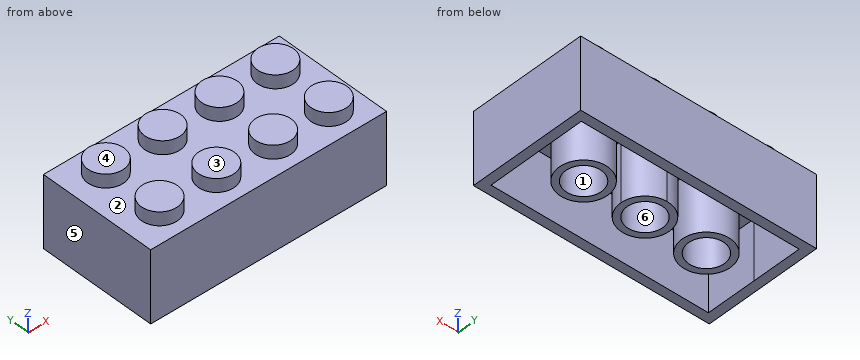
from build123d import *

# Parameters (mm, degrees)
F0_W     = 31.64
F0_H     = 15.74
F1_DEPTH = 9.59
F2_R     = 2.425
F3_DEPTH = 1.8
F5_DEPTH = 8


with BuildPart() as f1:
    # F0 (on Top) → F1 (new body)
    with BuildSketch(Plane.XY):
        with Locations((15.82, 7.87)):
            Rectangle(F0_W, F0_H)
    extrude(amount=F1_DEPTH)

    # F2 (on face) → F3 (join)
    with BuildSketch(Plane.XY.offset(9.59)):
        with Locations((4.7746349379, 11.815)):
            Circle(F2_R)
        with Locations((12.3955499551, 11.815)):
            Circle(F2_R)
        with Locations((20.0164649723, 11.815)):
            Circle(F2_R)
        with Locations((27.4894218309, 11.7763556091)):
            Circle(F2_R)
        with Locations((4.7746349379, 3.925)):
            Circle(F2_R)
        with Locations((12.3955499551, 3.925)):
            Circle(F2_R)
        with Locations((20.0164649723, 3.925)):
            Circle(F2_R)
        with Locations((27.4894218309, 3.925)):
            Circle(F2_R)
    extrude(amount=F3_DEPTH)

    # F4 (on face) → F5 (cut)
    with BuildSketch(Plane(origin=(0, 0, 0), x_dir=(1, 0, 0), z_dir=(0, 0, -1))):
        with BuildLine():
            ThreePointArc((19.07, -7.87), (18.1189275762, -10.1672662012), (15.8223495388, -11.1199991507))
            Line((15.8223495388, -11.1199991507), (15.8223495388, -14.52))
            Line((15.8223495388, -14.52), (30.4358961851, -14.52))
            Line((30.4358961851, -14.52), (30.4199965129, -7.87))
            Line((30.4199965129, -7.87), (27.31, -7.87))
            ThreePointArc((27.31, -7.87), (24.06, -11.12), (20.81, -7.87))
            Line((20.81, -7.87), (19.07, -7.87))
        make_face()
        with BuildLine():
            Line((15.817648704, -1.22), (15.817648704, -4.6200008506))
            ThreePointArc((15.817648704, -4.6200008506), (18.1172655798, -5.5710718028), (19.07, -7.87))
            Line((19.07, -7.87), (20.81, -7.87))
            ThreePointArc((20.81, -7.87), (24.06, -4.62), (27.31, -7.87))
            Line((27.31, -7.87), (30.4199965129, -7.87))
            Line((30.4199965129, -7.87), (30.4040968407, -1.22))
            Line((30.4040968407, -1.22), (15.817648704, -1.22))
        make_face()
        with BuildLine():
            ThreePointArc((4.33, -7.87), (7.58, -4.62), (10.83, -7.87))
            Line((10.83, -7.87), (12.57, -7.87))
            ThreePointArc((12.57, -7.87), (13.5210718028, -5.5727344202), (15.817648704, -4.6200008506))
            Line((15.817648704, -4.6200008506), (15.817648704, -1.22))
            Line((15.817648704, -1.22), (1.2312005673, -1.22))
            Line((1.2312005673, -1.22), (1.2200017299, -7.87))
            Line((1.2200017299, -7.87), (4.33, -7.87))
        make_face()
        with BuildLine():
            Line((12.57, -7.87), (10.83, -7.87))
            ThreePointArc((10.83, -7.87), (7.58, -11.12), (4.33, -7.87))
            Line((4.33, -7.87), (1.2200017299, -7.87))
            Line((1.2200017299, -7.87), (1.2088028926, -14.52))
            Line((1.2088028926, -14.52), (15.8223495388, -14.52))
            Line((15.8223495388, -14.52), (15.8223495388, -11.1199991507))
            ThreePointArc((15.8223495388, -11.1199991507), (13.5227337988, -10.1689275762), (12.57, -7.87))
        make_face()
        with BuildLine():
            Line((5.18, -7.87), (9.98, -7.87))
            ThreePointArc((9.98, -7.87), (7.58, -5.47), (5.18, -7.87))
        make_face()
        with BuildLine():
            ThreePointArc((5.18, -7.87), (7.58, -10.27), (9.98, -7.87))
            Line((9.98, -7.87), (5.18, -7.87))
        make_face()
        with BuildLine():
            Line((18.22, -7.87), (13.42, -7.87))
            ThreePointArc((13.42, -7.87), (15.82, -10.27), (18.22, -7.87))
        make_face()
        with BuildLine():
            ThreePointArc((18.22, -7.87), (15.82, -5.47), (13.42, -7.87))
            Line((13.42, -7.87), (18.22, -7.87))
        make_face()
        with BuildLine():
            ThreePointArc((26.46, -7.87), (24.06, -5.47), (21.66, -7.87))
            Line((21.66, -7.87), (26.46, -7.87))
        make_face()
        with BuildLine():
            Line((26.46, -7.87), (21.66, -7.87))
            ThreePointArc((21.66, -7.87), (24.06, -10.27), (26.46, -7.87))
        make_face()
    extrude(amount=-F5_DEPTH, mode=Mode.SUBTRACT)


solid = f1.part
Here's how the part is built. I have some questions about the finished solid (model axes, mm). Face numbers are marked on the shaded views. A direction names the side the tool comes from. Give positions to 0.01 mm unless a question says otherwise; leave off trailing zeros. Order: outer loops, then holes, each group sorted by start corner. A loop starts at its lowest first (then second) coordinate and runs counter-clockwise, first axis right, second up. Notation, with made-up numbers: (-16.75, 37) -> (30.25, 37) arc R16 ccw to (30.25, 41) -> close; hole circle Ø10 at (74.25, -10). An arc over 180 degrees is marked (long way). Use a Markdown table: item, result. Add a question column.
Item 1: If we mould it in two halves opening along X, with no side actions, what happens to the marked faces 4, 5 and 6? For each: pulls with the +X half, pulls with the -X half, needs draft (parallel to the pull), parting line crosses it, or undercut.
Item 2: I need wall thicknesses on line 1 (Y direction, x = 7.58, z = 5.75); line 2 (Y direction, x = 29, z = 1.75); line 3 (Y direction, x = 5, z = 0.5). Which ranges of each line are inside material? Lowest first, please.
Item 3: Imagine slicing it at C-C on y = 13. Please give me the cut outline in (x, z), plus the area to 3 significant figures.
Item 4: Will these pins go through, and if not, where does the flat tip stop? pin 1 (3 mm diameter, centred on x = 15.82, y = 7.87, fed in from +Z); pin 2 (2.5 mm diameter, centred on x = 8.5, y = 8, fed in from -Z).
Item 5: Imagine slicing it at B-B on x = 24.06. Please give me the cut outline in (y, z), plus the area to 3 significant figures.
Item 6: Imagine slicing it at A-A on z = 5.5. Please give me the cut outline in (x, y), plus the area to 3 significant figures.
Item 7: Imagine slicing it at D-D on x = 2. Please give me the cut outline in (y, z), plus the area to 3 significant figures.
Item 8: For the marked faces 1, 2 and 3, which set-ups out of +Z, -Z, +X, -X, +Y, -Y let a thin tool reach every point of the face, with its end or its side?
Data:
| question | item | result |
|---|---|---|
| 1 | face 4 | needs draft |
| 1 | face 5 | pulls with the -X half |
| 1 | face 6 | undercut |
| 2 | line 1 | y = 0 to 1.22, 4.62 to 5.47, 10.27 to 11.12, 14.52 to 15.74 |
| 2 | line 2 | y = 0 to 1.22, 14.52 to 15.74 |
| 2 | line 3 | y = 0 to 1.22, 5.89 to 9.85, 14.52 to 15.74 |
| 3 | outline | (0, 0) -> (1.21, 0) -> (1.21, 8) -> (30.43, 8) -> (30.43, 0) -> (31.64, 0) -> (31.64, 9.59) -> (29.58, 9.59) -> (29.58, 11.39) -> (25.4, 11.39) -> (25.4, 9.59) -> (22.13, 9.59) -> (22.13, 11.39) -> (17.9, 11.39) -> (17.9, 9.59) -> (14.51, 9.59) -> (14.51, 11.39) -> (10.28, 11.39) -> (10.28, 9.59) -> (6.89, 9.59) -> (6.89, 11.39) -> (2.66, 11.39) -> (2.66, 9.59) -> (0, 9.59) -> close |
| 3 | area | 100 mm² |
| 4 | pin 1 | stops at z = 9.59 |
| 4 | pin 2 | stops at z = 8 |
| 5 | outline | (0, 0) -> (1.22, 0) -> (1.22, 8) -> (4.62, 8) -> (4.62, 0) -> (5.47, 0) -> (5.47, 8) -> (10.27, 8) -> (10.27, 0) -> (11.12, 0) -> (11.12, 8) -> (14.52, 8) -> (14.52, 0) -> (15.74, 0) -> (15.74, 9.59) -> (0, 9.59) -> close |
| 5 | area | 58.1 mm² |
| 6 | outline | (0, 0) -> (31.64, 0) -> (31.64, 15.74) -> (0, 15.74) -> close; circle Ø6.5 at (7.58, 7.87); circle Ø6.5 at (15.82, 7.87); circle Ø6.5 at (24.06, 7.87); hole (1.21, 14.52) -> (1.23, 1.22) -> (30.4, 1.22) -> (30.44, 14.52) -> close; hole circle Ø4.8 at (7.58, 7.87); hole circle Ø4.8 at (15.82, 7.87); hole circle Ø4.8 at (24.06, 7.87) |
| 6 | area | 155 mm² |
| 7 | outline | (0, 0) -> (1.22, 0) -> (1.22, 8) -> (14.52, 8) -> (14.52, 0) -> (15.74, 0) -> (15.74, 9.59) -> (0, 9.59) -> close |
| 7 | area | 44.5 mm² |
| 8 | face 1 | -Z |
| 8 | face 2 | +Z |
| 8 | face 3 | +Z, +X, -X, +Y, -Y |
